from build123d import *

# Parameters (mm, degrees)
BOSS_EXTRUDE1_DEPTH = 6.35
SKETCH2_R           = 2
CUT_EXTRUDE1_DEPTH  = 37.477972806
SKETCH3_R           = 2
CUT_EXTRUDE2_DEPTH  = 37.477972806
FILLET1_R           = 1.27


with BuildPart() as part:
    # Sketch1 → Boss-Extrude1 (new body)
    with BuildSketch(Plane.XY):
        Polygon((0, 0), (6.35, 0), (6.35, 19.05), (25.4, 19.05), (25.4, 25.4), (0, 25.4), align=None)
    extrude(amount=BOSS_EXTRUDE1_DEPTH)

    # Sketch2 → Cut-Extrude1 (cut, through all)
    with BuildSketch(Plane(origin=(0, 25.4, 0), x_dir=(1, 0, 0), z_dir=(0, 1, 0))):
        with Locations(Location((21.59, -3.175, 0), (0, 0, 270))):
            Circle(SKETCH2_R)
    extrude(amount=-CUT_EXTRUDE1_DEPTH, mode=Mode.SUBTRACT)

    # Sketch3 → Cut-Extrude2 (cut, through all)
    with BuildSketch(Plane.ZY):
        with Locations((3.175, 3.81)):
            Circle(SKETCH3_R)
    extrude(amount=-CUT_EXTRUDE2_DEPTH, mode=Mode.SUBTRACT)

    # Fillet1
    # the kernel refuses this fillet: 1.27 mm, written as the material it takes off along each edge
    with BuildSketch(Plane(origin=(1.27, 24.13, 1.27), x_dir=(0, 0, -1), z_dir=(-1, 0, 0))) as fillet1_piece_1_section:
        Polygon((0, 0), (FILLET1_R, 0), (FILLET1_R, -FILLET1_R), (0, -FILLET1_R), align=None)
    fillet1_piece_1 = extrude(amount=FILLET1_R, mode=Mode.PRIVATE)
    fillet1_piece_1 = fillet1_piece_1 - Plane(origin=(1.27, 24.13, 1.27), x_dir=(0, -0.7071067811865475, 0.7071067811865475), z_dir=(-1, 0, 0)) * Sphere(FILLET1_R, mode=Mode.PRIVATE)
    add(fillet1_piece_1, mode=Mode.SUBTRACT)
    with BuildSketch(Plane(origin=(1.27, 24.13, 5.08), x_dir=(0, 0, 1), z_dir=(-1, 0, 0))) as fillet1_piece_2_section:
        Polygon((0, 0), (FILLET1_R, 0), (FILLET1_R, FILLET1_R), (0, FILLET1_R), align=None)
    fillet1_piece_2 = extrude(amount=FILLET1_R, mode=Mode.PRIVATE)
    fillet1_piece_2 = fillet1_piece_2 - Plane(origin=(1.27, 24.13, 5.08), x_dir=(0, -0.7071067811865475, -0.7071067811865475), z_dir=(-1, 0, 0)) * Sphere(FILLET1_R, mode=Mode.PRIVATE)
    add(fillet1_piece_2, mode=Mode.SUBTRACT)
    with BuildSketch(Plane(origin=(24.13, 24.13, 1.27), x_dir=(0, 0, -1), z_dir=(1, 0, 0))) as fillet1_piece_3_section:
        Polygon((0, 0), (FILLET1_R, 0), (FILLET1_R, FILLET1_R), (0, FILLET1_R), align=None)
    fillet1_piece_3 = extrude(amount=FILLET1_R, mode=Mode.PRIVATE)
    fillet1_piece_3 = fillet1_piece_3 - Plane(origin=(24.13, 24.13, 1.27), x_dir=(0, -0.7071067811865475, 0.7071067811865475), z_dir=(1, 0, 0)) * Sphere(FILLET1_R, mode=Mode.PRIVATE)
    add(fillet1_piece_3, mode=Mode.SUBTRACT)
    with BuildSketch(Plane(origin=(24.13, 24.13, 5.08), x_dir=(0, 0, 1), z_dir=(1, 0, 0))) as fillet1_piece_4_section:
        Polygon((0, 0), (FILLET1_R, 0), (FILLET1_R, -FILLET1_R), (0, -FILLET1_R), align=None)
    fillet1_piece_4 = extrude(amount=FILLET1_R, mode=Mode.PRIVATE)
    fillet1_piece_4 = fillet1_piece_4 - Plane(origin=(24.13, 24.13, 5.08), x_dir=(0, -0.7071067811865475, -0.7071067811865475), z_dir=(1, 0, 0)) * Sphere(FILLET1_R, mode=Mode.PRIVATE)
    add(fillet1_piece_4, mode=Mode.SUBTRACT)
    with BuildSketch(Plane(origin=(1.27, 1.27, 1.27), x_dir=(-1, 0, 0), z_dir=(0, -1, 0))) as fillet1_piece_5_section:
        Polygon((0, 0), (FILLET1_R, 0), (FILLET1_R, FILLET1_R), (0, FILLET1_R), align=None)
    fillet1_piece_5 = extrude(amount=FILLET1_R, mode=Mode.PRIVATE)
    fillet1_piece_5 = fillet1_piece_5 - Plane(origin=(1.27, 1.27, 1.27), x_dir=(0.7071067811865475, 0, 0.7071067811865475), z_dir=(0, -1, 0)) * Sphere(FILLET1_R, mode=Mode.PRIVATE)
    add(fillet1_piece_5, mode=Mode.SUBTRACT)
    with BuildSketch(Plane(origin=(1.27, 1.27, 5.08), x_dir=(-1, 0, 0), z_dir=(0, -1, 0))) as fillet1_piece_6_section:
        Polygon((0, 0), (FILLET1_R, 0), (FILLET1_R, -FILLET1_R), (0, -FILLET1_R), align=None)
    fillet1_piece_6 = extrude(amount=FILLET1_R, mode=Mode.PRIVATE)
    fillet1_piece_6 = fillet1_piece_6 - Plane(origin=(1.27, 1.27, 5.08), x_dir=(0.7071067811865475, 0, -0.7071067811865475), z_dir=(0, -1, 0)) * Sphere(FILLET1_R, mode=Mode.PRIVATE)
    add(fillet1_piece_6, mode=Mode.SUBTRACT)
    with BuildSketch(Plane(origin=(0, 25.4, 1.27), x_dir=(0, -1, 0), z_dir=(0, 0, 1)), Plane(origin=(25.4, 25.4, 1.27), x_dir=(-1, 0, 0), z_dir=(0, 0, 1)), Plane(origin=(0, 0, 1.27), x_dir=(1, 0, 0), z_dir=(0, 0, 1))) as fillet1_piece_7:
        with BuildLine():
            CenterArc((FILLET1_R, FILLET1_R), FILLET1_R, 180, 90)
            Line((0, FILLET1_R), (0, 0))
            Line((0, 0), (FILLET1_R, 0))
        make_face()
    extrude(amount=3.81, mode=Mode.SUBTRACT)
    with BuildSketch(Plane(origin=(25.4, 15.875, 6.35), x_dir=(-1, 0, 0), z_dir=(0, 1, 0)), Plane(origin=(1.27, 0, 0), x_dir=(0, 0, 1), z_dir=(1, 0, 0))) as fillet1_piece_8:
        with BuildLine():
            CenterArc((FILLET1_R, -FILLET1_R), FILLET1_R, 90, 90)
            Line((0, -FILLET1_R), (0, 0))
            Line((0, 0), (FILLET1_R, 0))
        make_face()
    extrude(amount=8.255, mode=Mode.SUBTRACT)
    with BuildSketch(Plane(origin=(24.13, 25.4, 6.35), x_dir=(0, -1, 0), z_dir=(-1, 0, 0)), Plane(origin=(0, 24.13, 0), x_dir=(0, 0, 1), z_dir=(0, -1, 0))) as fillet1_piece_9:
        with BuildLine():
            CenterArc((FILLET1_R, -FILLET1_R), FILLET1_R, 90, 90)
            Line((0, -FILLET1_R), (0, 0))
            Line((0, 0), (FILLET1_R, 0))
        make_face()
    extrude(amount=22.86, mode=Mode.SUBTRACT)
    with BuildSketch(Plane(origin=(0, 24.13, 6.35), x_dir=(0, 0, -1), z_dir=(0, -1, 0)), Plane(origin=(24.13, 25.4, 0), x_dir=(0, -1, 0), z_dir=(-1, 0, 0))) as fillet1_piece_10:
        with BuildLine():
            CenterArc((FILLET1_R, FILLET1_R), FILLET1_R, 180, 90)
            Line((0, FILLET1_R), (0, 0))
            Line((0, 0), (FILLET1_R, 0))
        make_face()
    extrude(amount=22.86, mode=Mode.SUBTRACT)
    with BuildSketch(Plane(origin=(25.4, 15.875, 0), x_dir=(-1, 0, 0), z_dir=(0, 1, 0)), Plane(origin=(1.27, 0, 6.35), x_dir=(0, 0, -1), z_dir=(1, 0, 0))) as fillet1_piece_11:
        with BuildLine():
            CenterArc((FILLET1_R, FILLET1_R), FILLET1_R, 180, 90)
            Line((0, FILLET1_R), (0, 0))
            Line((0, 0), (FILLET1_R, 0))
        make_face()
    extrude(amount=8.255, mode=Mode.SUBTRACT)


solid = part.part
Verification items for the finished model (mm, model axes). A direction names the side the tool comes from. Round coordinates to 2 decimals unless told otherwise and drop trailing zeros. Write each loop counter-clockwise with the first axis right and the second up, starting at its lowest first coordinate (ties: lowest second). Pieces come first, ordered by that corner, then holes.
(1) Section check C-C (y = 21). Enter the section's corners in (x, z) (3 decimals).
Returned:
outline: (0, 1.27) arc R1.27 ccw to (1.27, 0) - (24.13, 0) arc R1.27 ccw to (25.4, 1.27) - (25.4, 5.08) arc R1.27 ccw to (24.13, 6.35) - (1.27, 6.35) arc R1.27 ccw to (0, 5.08) - close; hole circle Ø4 at (21.59, 3.175)
(2) Mould release check, pull along X, two halves, no side actions. Record for faces 1 (the cylindrical face through (19.638, 22.269, 2.741)), 2 (the flat face through (7, 20, 6.35)), 3 (the cylindrical face through (0.362, 0.382, 3.148)): pulls with the +X half, pulls with the -X half, needs draft (parallel to the pull), parting line crosses it, or undercut.
Returned:
face 1: undercut
face 2: needs draft
face 3: pulls with the -X half
(3) Material ranges on line 1 (Z direction, x = 3.5, y = 3.81) (3 decimals); line 2 (Y direction, x = 24, z = 2), recorded low to high.
Returned:
line 1: z = 0 to 1.175, 5.175 to 6.35
line 2: y = 19.05 to 25.4
(4) Section check D-D (x = 21.59). Enter the section's corners in (y, z) (3 decimals), plus the area to 3 significant figures.
Returned:
outline: (19.05, 0) - (24.13, 0) arc R1.27 ccw to (25.396, 1.175) - (19.05, 1.175) - close; (19.05, 5.175) - (25.396, 5.175) arc R1.27 ccw to (24.13, 6.35) - (19.05, 6.35) - close
area: 14.2 mm2
(5) Access from +Z, -Z, +X, -X, +Y, -Y to the whole of each face (thin tool, end or side, straight path). Record for faces 4 (the cylindrical face through (3.774, 0.362, 0.382)), 5 (the flat face through (6.35, 9, 3)).
Returned:
face 4: -Z, +X, -X, -Y
face 5: +Z, -Z, +X, -Y
(6) Depth check by flat-ended pin: pin 1 Ø3 at (x, z) = (9.5, 3.5) entering from -Y; pin 2 Ø3 at (y, z) = (9.5, 4.5) entering from +X; pin 3 Ø5 at (x, y) = (11, 15) entering from +Z. Enter the tip coordinate at first touch or a pass-through.
Returned:
pin 1: stops at y = 19.05
pin 2: stops at x = 6.35
pin 3: passes through
(7) Section check B-B (z = 2.25). Enter the section's corners in (x, y).
Returned:
outline: (0, 1.27) arc R1.27 ccw to (1.27, 0) - (6.35, 0) - (6.35, 2.04) - (0, 2.04) - close; (0, 5.58) - (6.35, 5.58) - (6.35, 19.05) - (19.82, 19.05) - (19.82, 25.4) - (1.27, 25.4) arc R1.27 ccw to (0, 24.13) - close; (23.36, 19.05) - (25.4, 19.05) - (25.4, 24.13) arc R1.27 ccw to (24.13, 25.4) - (23.36, 25.4) - close
(8) Section check A-A (x = 2.25). Enter the section's corners in (y, z) (3 decimals), plus the area to 3 significant figures.
Returned:
outline: (0, 1.27) arc R1.27 ccw to (1.27, 0) - (24.13, 0) arc R1.27 ccw to (25.4, 1.27) - (25.4, 5.08) arc R1.27 ccw to (24.13, 6.35) - (1.27, 6.35) arc R1.27 ccw to (0, 5.08) - close; hole circle Ø4 at (3.81, 3.175)
area: 147 mm2
